The listing builds one solid part. Answer for the finished solid, in the listing's coordinates (mm). Coordinates: 2 decimals unless noted, no trailing zeros. Order: outer loops, then holes, each group sorted by start corner. A loop starts at its lowest first (then second) coordinate and runs counter-clockwise, first axis right, second up. Notation, with made-up numbers: (-38, 0) -> (14, 0) arc R18 ccw to (14, 23) -> close; hole circle Ø9 at (-29.75, 71.5). An arc over 180 degrees is marked (long way). Answer in a Markdown table with one row per item.
```python
from build123d import *

# Parameters (mm, degrees)
BOSS_EXTRUDE1_OUTLINE_R = 21.1
BOSS_EXTRUDE1_DEPTH     = 25


# Read off the part's stored shape, not the designer's step: Boss-Extrude1
with BuildPart() as part:
    # Boss-Extrude1 outline → Boss-Extrude1 (new body)
    with BuildSketch(Plane.XY.offset(29)):
        Circle(BOSS_EXTRUDE1_OUTLINE_R)
    extrude(amount=BOSS_EXTRUDE1_DEPTH)


solid = part.part
```
(1) Find the intervals of material crossed by line 1 along Y through (x, z) = (0, 31.25); line 2 along X through (y, z) = (-9, 36.5); line 3 along Y through (x, z) = (-13, 30.5), in increasing order. Write a range as from..to.
Check values:
| item | result |
|---|---|
| line 1 | -21.1..21.1 |
| line 2 | -19.08..19.08 |
| line 3 | -16.62..16.62 |
(2) Flat-ended cylindrical pins translate along their axes: pin 1 (10 mm diameter, centred on x = -12, z = 38.5, fed in from +Y) (3 decimals); pin 2 (5 mm diameter, centred on y = -15.5, z = 45, fed in from -X); pin 3 (10 mm diameter, centred on x = 8.5, z = 42.5, fed in from +Y). Find the tip coordinate at first contact, or state that the pin passes through.
Check values:
| item | result |
|---|---|
| pin 1 | y = 19.905 |
| pin 2 | x = -16.62 |
| pin 3 | y = 20.81 |
(3) A cutting plane is placed at A-A, the plane x = -13. Determine the outline of the cut face in (y, z).
Check values:
| item | result |
|---|---|
| outline | (-16.62, 29) -> (16.62, 29) -> (16.62, 54) -> (-16.62, 54) -> close |
(4) A cutting plane is placed at B-B, the plane z = 36. Determine the outline of the cut face in (x, y), then the cut area to 3 significant figures.
Check values:
| item | result |
|---|---|
| outline | circle Ø42.2 at (0, 0) |
| area | 1,400 mm² |
(5) A cutting plane is placed at C-C, the plane y = -17.5. Determine the outline of the cut face in (x, z).
Check values:
| item | result |
|---|---|
| outline | (-11.79, 29) -> (11.79, 29) -> (11.79, 54) -> (-11.79, 54) -> close |
